Study the drawing (mm; zero at the part's minimum x, y, z) and answer. A direction names the side the tool comes from. Round coordinates to 2 decimals unless told otherwise and drop trailing zeros. Write each loop counter-clockwise with the first axis right and the second up, starting at its lowest first coordinate (ties: lowest second). Pieces come first, ordered by that corner, then holes.
(1) A cutting plane is placed at C-C, the plane z = 8.5. Give the vertices of the cut face in (x, y).
(2) Each of these flat-tipped pins is pushed along its axis until it touches: pin 1 Ø5 at (y, z) = (5, 7) entering from +X; pin 2 Ø1.5 at (y, z) = (4.5, 3.5) entering from +X (1 decimal); pin 3 Ø6 at (x, z) = (11.5, 9) entering from -Y. Where does it stop, or does it pass through?
(3) A cutting plane is placed at D-D, the plane y = 11.5. Give the vertices of the cut face in (x, z).
(4) The mould has two halves that part along Y. Classify the marked faces 1, 2 and 3: +Y half, -Y half, draft (parallel to the pull), parting line (faces both ways), or undercut.
(5) A cutting plane is placed at B-B, the plane y = 27. Give the vertices of the cut face in (x, z) (1 decimal).
(6) A cutting plane is placed at A-A, the plane x = 29.5. Give the vertices of the cut face in (y, z).
(7) Find the intervals of material crossed by probe 1 along X at (y, z) = (25, 6.25); probe 2 along X at (y, z) = (24.5, 7.5); probe 3 along Y at (x, z) = (17, 3), in increasing order.
(8) For the marked faces 4, 5, 6, 7 and 8, determine the directions among +Z, -Z, +X, -X, +Y, -Y from which every point of the face is accessible in a straight line to the end or side of a thin tool.
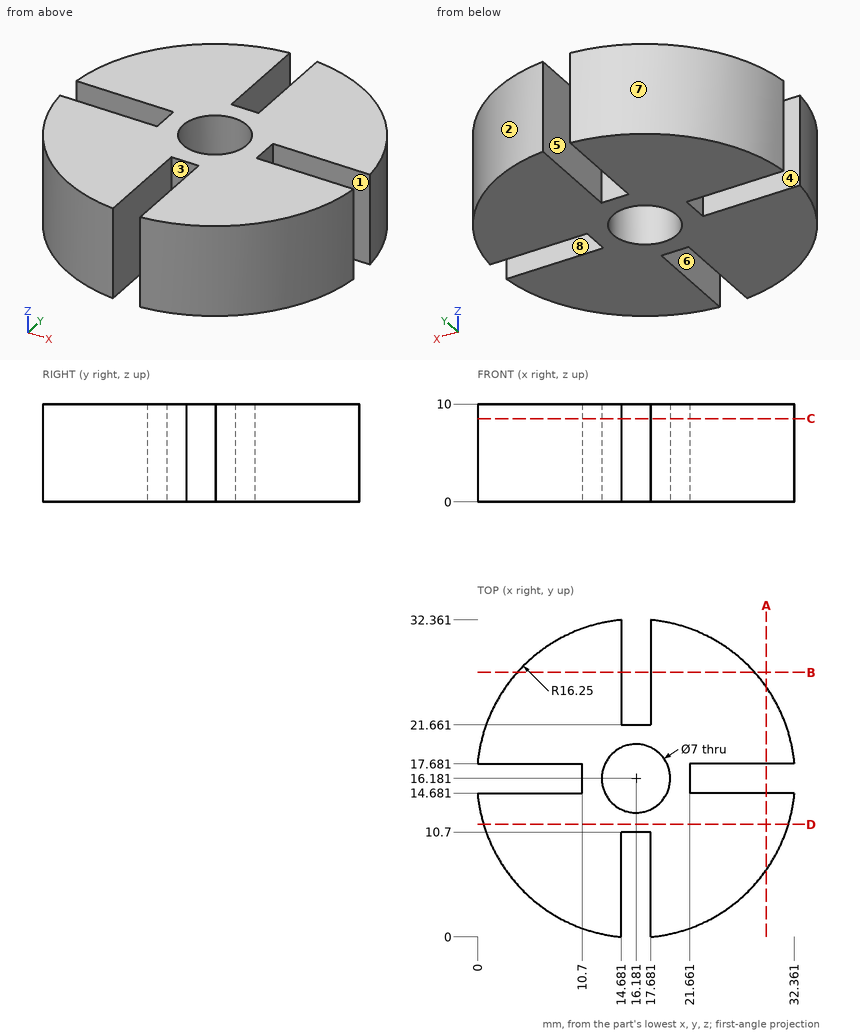
Solutions:
1. outline: (0, 14.68) arc R16.25 ccw to (14.68, 0) - (14.68, 10.7) - (17.68, 10.7) - (17.68, 0) arc R16.25 ccw to (32.36, 14.68) - (21.66, 14.68) - (21.66, 17.68) - (32.36, 17.68) arc R16.25 ccw to (17.68, 32.36) - (17.68, 21.66) - (14.68, 21.66) - (14.68, 32.36) arc R16.25 ccw to (0, 17.68) - (10.7, 17.68) - (10.7, 14.68) - close; hole circle Ø7 at (16.18, 16.18)
2. pin 1: stops at x = 29.92
2. pin 2: stops at x = 28.2
2. pin 3: stops at y = 0.02
3. outline: (0.62, 0) - (31.74, 0) - (31.74, 10) - (0.62, 10) - close
4. face 1: undercut
4. face 2: +Y half
4. face 3: -Y half
5. outline: (4.1, 0) - (14.7, 0) - (14.7, 10) - (4.1, 10) - close; (17.7, 0) - (28.3, 0) - (28.3, 10) - (17.7, 10) - close
6. outline: (6.87, 0) - (14.68, 0) - (14.68, 10) - (6.87, 10) - close; (17.68, 0) - (25.49, 0) - (25.49, 10) - (17.68, 10) - close
7. probe 1: x = 2.53 to 14.68, 17.68 to 29.83
7. probe 2: x = 2.22 to 14.68, 17.68 to 30.14
7. probe 3: y = 10.7 to 12.78, 19.58 to 21.66
8. face 4: +Z, -Z, -X
8. face 5: +Z, -Z, +Y
8. face 6: +Z, -Z, -Y
8. face 7: +Z, -Z, -X, +Y
8. face 8: +Z, -Z, +X
